Verification items for the finished model (mm, model axes). A direction names the side the tool comes from. Give positions to 0.01 mm unless a question says otherwise; leave off trailing zeros. Loops run counter-clockwise (first coordinate to the right, second up) from the corner with the lowest first, then second, coordinate; pieces in that order, holes last. Notation, with made-up numbers: M -9.75,62.5 L 15.25,62.5 A22 ccw 15.25,77.5 Z; hole C 56,86 d5. An arc over 180 degrees is marked long. Use CSV: the item, a comma, the result in double quotes.
from build123d import *

# Parameters (mm, degrees)
F1_DEPTH = 20
F2_DEPTH = 2
F3_SIZE  = 1.4
F4_R     = 1


with BuildPart() as f1:
    # F0 (on Front) → F1 (new body)
    with BuildSketch(Plane.XZ):
        with BuildLine():
            Line((-28.994949, 28.994949), (-2.828427, 2.828427))
            ThreePointArc((-2.828427, 2.828427), (0, 1.656854), (2.828427, 2.828427))
            Line((2.828427, 2.828427), (28.994949, 28.994949))
            ThreePointArc((28.994949, 28.994949), (29.600194, 57.358261), (1.28852, 59.172891))
            ThreePointArc((1.28852, 59.172891), (0, 58.702505), (-1.28852, 59.172891))
            ThreePointArc((-1.28852, 59.172891), (-29.600194, 57.358261), (-28.994949, 28.994949))
        make_face()
        with BuildLine():
            ThreePointArc((1.59099, 4.065864), (0, 3.406854), (-1.59099, 4.065864))
            Line((-1.59099, 4.065864), (-27.757512, 30.232386))
            ThreePointArc((-27.757512, 30.232386), (-28.311096, 56.174738), (-2.415975, 57.83448))
            ThreePointArc((-2.415975, 57.83448), (0, 56.952505), (2.415975, 57.83448))
            ThreePointArc((2.415975, 57.83448), (28.311096, 56.174738), (27.757512, 30.232386))
            Line((27.757512, 30.232386), (1.59099, 4.065864))
        make_face(mode=Mode.SUBTRACT)
    extrude(amount=F1_DEPTH)

    # F0 (on Front) → F2 (join)
    with BuildSketch(Plane.XZ):
        with BuildLine():
            ThreePointArc((-6.363961, -0.707107), (0, -3.343146), (6.363961, -0.707107))
            Line((6.363961, -0.707107), (32.530483, 25.459415))
            ThreePointArc((32.530483, 25.459415), (34.084411, 59.824317), (0, 64.473416))
            ThreePointArc((0, 64.473416), (-34.084411, 59.824317), (-32.530483, 25.459415))
            Line((-32.530483, 25.459415), (-6.363961, -0.707107))
        make_face()
        with BuildLine():
            ThreePointArc((2.828427, 2.828427), (0, 1.656854), (-2.828427, 2.828427))
            Line((-2.828427, 2.828427), (-28.994949, 28.994949))
            ThreePointArc((-28.994949, 28.994949), (-29.600194, 57.358261), (-1.28852, 59.172891))
            ThreePointArc((-1.28852, 59.172891), (0, 58.702505), (1.28852, 59.172891))
            ThreePointArc((1.28852, 59.172891), (29.600194, 57.358261), (28.994949, 28.994949))
            Line((28.994949, 28.994949), (2.828427, 2.828427))
        make_face(mode=Mode.SUBTRACT)
    extrude(amount=F2_DEPTH)

    # F3
    f3_edges = [f1.edges().sort_by_distance(p)[0] for p in [
        (15.911688, -20, 15.911688),
    ]]
    chamfer(f3_edges, length=F3_SIZE)

    # F4
    f4_edges = [f1.edges().sort_by_distance(p)[0] for p in [
        (15.911688, -2, 15.911688),
        (19.447222, -2, 12.376154),
    ]]
    fillet(f4_edges, radius=F4_R)


solid = f1.part
(1) Tool access check on faces 1 (the cylindrical face through (-0.037, -9.86, 56.953)), 2 (the cylindrical face through (0.02, -10.691, 58.703)), 3 (the flat face through (16, -11, 16)). Record the directions out of +Z, -Z, +X, -X, +Y, -Y that give a thin tool (end or side, any length) a straight path to the whole face; none if there is none.
Calculated:
face 1,"+Y, -Y"
face 2,"+Z, -Y"
face 3,"-Z, +X, -Y"
(2) Depth check by flat-ended pin: pin 1 Ø2 at (x, y) = (16, -14.5) entering from +Z; pin 2 Ø12 at (x, y) = (3, -8.5) entering from +Z; pin 3 Ø6 at (y, z) = (-16, 30.5) entering from -X. Enter the tip coordinate at first touch or a pass-through.
Calculated:
pin 1,"stops at z = 63.99"
pin 2,"stops at z = 63.24"
pin 3,"stops at x = -32.4"
(3) Scan lines: L1, parallel to X at y = -8, z = 57.5; L2, parallel to X at y = -1, z = 58; L3, parallel to Y at x = 34, z = 34. Record each from-to range of solid material in increasing order. Write a range as from..to.
Calculated:
L1,"x = -29.47..-26.97, -1.95..1.95, 26.97..29.47"
L2,"x = -35.47..-26.38, -2.62..2.62, 26.38..35.47"
L3,"y = -2..0"
(4) Mould release check, pull along X, two halves, no side actions. Record for faces 4 (the flat face through (19.26, -0.49, 12.19)), 5 (the flat face through (-16, -11, 16)), 6 (the cylindrical face through (28.037, -9.86, 56.467)): released by +X, released by -X, zero draft, split by the parting line, or undercut.
Calculated:
face 4,"released by +X"
face 5,"released by -X"
face 6,"undercut"
(5) Section check A-A on y = -6. Record the cut outline in (x, z).
Calculated:
outline,"M -28.99,28.99 L -2.83,2.83 A4 ccw 2.83,2.83 L 28.99,28.99 A20.5 ccw 1.29,59.17 A2 cw -1.29,59.17 A20.5 ccw Z; hole M -27.76,30.23 L -1.59,4.07 A2.25 ccw 1.59,4.07 L 27.76,30.23 A18.75 ccw 2.42,57.83 A3.75 cw -2.42,57.83 A18.75 ccw Z"
